Autodesk Inventor part; units mm, degrees
ref_plane "YZ Plane" through (0, 0, 0) normal (1, 0, 0) x (0, 1, 0)
ref_plane "XZ Plane" through (0, 0, 0) normal (0, 1, 0) x (-1, 0, 0)
ref_plane "XY Plane" through (0, 0, 0) normal (0, 0, 1) x (1, 0, 0)
sketch "Sketch1" plane through (0, 0, 0) normal (0, 1, 0) x (-1, 0, 0)
  circle A0 centre (0, 0) radius 10
  dimension "d0" = 20
extrude "Extrusion1" add sketch "Sketch1" along normal blind 30
sketch "Sketch2" plane through (0, 30, 0) normal (0, 1, 0) x (1, 0, 0)
  circle A0 centre (0, 0) radius 12.5
  dimension "d3" = 25
extrude "Extrusion2" add sketch "Sketch2" against normal blind 5
sketch "Sketch3" plane through (0, 30, 0) normal (0, 1, 0) x (1, 0, 0)
  circle A0 centre (0, 0) radius 7.5
  dimension "d7" = 15
extrude "Extrusion3" cut sketch "Sketch3" against normal blind 27
sketch "Sketch5" plane through (0, 0, 0) normal (0, -1, 0) x (1, 0, 0)
  circle A0 centre (0, 0) radius 5 construction
  circle A1 centre (0, 5) radius 1.5
  circle A2 centre (0, 0) radius 5 construction
  circle A3 centre (-4.3301, 2.5) radius 1.5
  circle A4 centre (0, 0) radius 5 construction
  circle A5 centre (-4.3301, -2.5) radius 1.5
  circle A6 centre (0, 0) radius 5 construction
  circle A7 centre (0, -5) radius 1.5
  circle A8 centre (0, 0) radius 5 construction
  circle A9 centre (4.3301, -2.5) radius 1.5
  circle A10 centre (0, 0) radius 5 construction
  circle A11 centre (4.3301, 2.5) radius 1.5
  circle A12 centre (0, 0) radius 1.5
  dimension "d32" = 10
  dimension "d33" = 3
  dimension "d36" = 360
  dimension "d38" = 3
extrude "Extrusion6" cut sketch "Sketch5" against normal blind 10
sketch "Sketch6" plane through (0, 30, 0) normal (0, 1, 0) x (1, 0, 0)
  point P0 (0, 0)
properties part number "DiffusionModule" material "ABS Plastic"
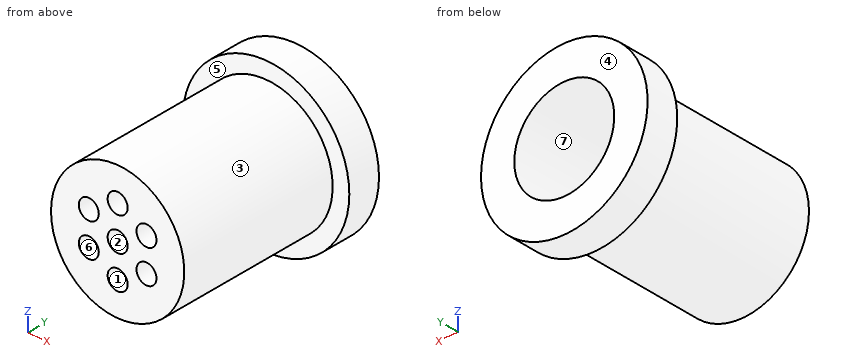
Work out the finished part from the listing and answer in its coordinate system (mm). Face numbers are marked on the shaded views. A direction names the side the tool comes from. Round coordinates to 2 decimals unless told otherwise and drop trailing zeros. Order: outer loops, then holes, each group sorted by start corner. A loop starts at its lowest first (then second) coordinate and runs counter-clockwise, first axis right, second up.
Q1. A cutting plane is placed at D-D, the plane z = -2.5. Determine the outline of the cut face in (x, y).
Solution:
outline: (-12.25, 25) - (-9.68, 25) - (-9.68, 0) - (-5.83, 0) - (-5.83, 3) - (-7.07, 3) - (-7.07, 30) - (-12.25, 30) - close; (-2.83, 0) - (2.83, 0) - (2.83, 3) - (-2.83, 3) - close; (5.83, 0) - (9.68, 0) - (9.68, 25) - (12.25, 25) - (12.25, 30) - (7.07, 30) - (7.07, 3) - (5.83, 3) - close
Q2. A tool of negligible diameter and unlimited length cuts with its end or side. For the marked faces 5, 6 and 7, from which of +Z, -Z, +X, -X, +Y, -Y can it reach the whole face along a straight path? Write none if from no direction.
Solution:
face 5: -Y
face 6: +Y, -Y
face 7: +Y
Q3. A cutting plane is placed at B-B, the plane z = 0. Determine the outline of the cut face in (x, y), then the cut area to 3 significant figures.
Solution:
outline: (-12.5, 25) - (-10, 25) - (-10, 0) - (-1.5, 0) - (-1.5, 3) - (-7.5, 3) - (-7.5, 30) - (-12.5, 30) - close; (1.5, 0) - (10, 0) - (10, 25) - (12.5, 25) - (12.5, 30) - (7.5, 30) - (7.5, 3) - (1.5, 3) - close
area: 211 mm2
Q4. The mould has two halves that part along X. Classify the marked faces 1, 2, 3 and 4: pulls with the +X half, pulls with the -X half, needs draft (parallel to the pull), parting line crosses it, or undercut.
Solution:
face 1: undercut
face 2: undercut
face 3: parting line crosses it
face 4: needs draft
Q5. Find the intervals of material crossed by line 1 along Z through (x, y) = (0, 1.45); line 2 along X through (y, z) = (7.25, -0.5); line 3 along Y through (x, z) = (-6.25, 9.75), in increasing order.
Solution:
line 1: z = -10 to -6.5, -3.5 to -1.5, 1.5 to 3.5, 6.5 to 10
line 2: x = -9.99 to -7.48, 7.48 to 9.99
line 3: y = 25 to 30
Q6. Given pin 1 Ø1.5 at (y, z) = (14.5, -4) entering from -X; pin 2 Ø1.8 at (x, z) = (-4.33, -2.5) entering from -Y; pin 3 Ø8 at (x, y) = (0, 17.5) entering from +Z; pin 4 Ø3 at (y, z) = (10.5, 3) entering from +X, each flat-ended and moving along its own axis, determine where each tip first touches the part or whether it passes through.
Solution:
pin 1: stops at x = -9.46
pin 2: passes through
pin 3: stops at z = 10
pin 4: stops at x = 9.89
Q7. A cutting plane is placed at C-C, the plane x = -4. Determine the outline of the cut face in (y, z), then the cut area to 3 significant figures.
Solution:
outline: (0, -9.17) - (25, -9.17) - (25, -11.84) - (30, -11.84) - (30, -6.34) - (3, -6.34) - (3, -3.96) - (0, -3.96) - close; (0, -1.04) - (3, -1.04) - (3, 1.04) - (0, 1.04) - close; (0, 3.96) - (3, 3.96) - (3, 6.34) - (30, 6.34) - (30, 11.84) - (25, 11.84) - (25, 9.17) - (0, 9.17) - close
area: 217 mm2
Q8. A cutting plane is placed at A-A, the plane x = 0. Determine the outline of the cut face in (y, z).
Solution:
outline: (0, -10) - (25, -10) - (25, -12.5) - (30, -12.5) - (30, -7.5) - (3, -7.5) - (3, -6.5) - (0, -6.5) - close; (0, -3.5) - (3, -3.5) - (3, -1.5) - (0, -1.5) - close; (0, 1.5) - (3, 1.5) - (3, 3.5) - (0, 3.5) - close; (0, 6.5) - (3, 6.5) - (3, 7.5) - (30, 7.5) - (30, 12.5) - (25, 12.5) - (25, 10) - (0, 10) - close
